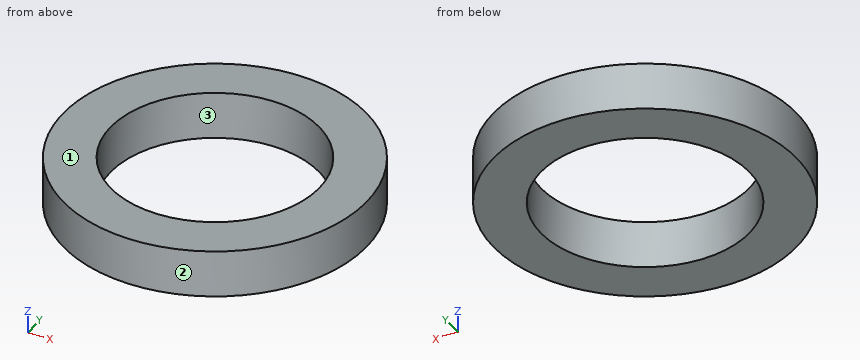
```python
from build123d import *

# Parameters (mm, degrees)
SKETCH1_R                = 2
BOSS_EXTRUDE1_DEPTH      = 6.35
CUT_EXTRUDE1_DEPTH       = 93.473426076
CUT_EXTRUDE1_DEPTH_BACK  = 93.473426076
SKETCH2_R                = 7
BOSS_EXTRUDE2_DEPTH      = 31.75
BOSS_EXTRUDE2_DEPTH_BACK = 12.7
SKETCH5_R                = 7
SKETCH6_R                = 7
BOSS_EXTRUDE3_DEPTH      = 6.35
FILLET1_R                = 6.35
FILLET2_R                = 3.175
SKETCH7_R                = 10.175
SKETCH7_R_2              = 7
BOSS_EXTRUDE4_DEPTH      = 3.175


with BuildPart() as part:
    # Sketch1 → Boss-Extrude1 (new, symmetric)
    # profile 1 of 3: a face of its own
    with BuildSketch(Plane.XY):
        Polygon((22.188571811, 51.670547503), (22.188571811, 37.229452497), (13.9055, 25.4), (13.9055, 0), (52.0055, 0), (52.0055, 25.4), (26.6055, 76.2), (13.9055, 76.2), (13.9055, 63.5), align=None)
        with Locations((33.493, 8.8)):
            Circle(SKETCH1_R, mode=Mode.SUBTRACT)
        with Locations((17.493, 8.8)):
            Circle(SKETCH1_R, mode=Mode.SUBTRACT)
    # profile 2 of 3: a face of its own
    with BuildSketch(Plane.XY):
        with Locations((17.493, 8.8)):
            Circle(SKETCH1_R)
    # profile 3 of 3: a face of its own
    with BuildSketch(Plane.XY):
        with Locations((33.493, 8.8)):
            Circle(SKETCH1_R)
    extrude(amount=BOSS_EXTRUDE1_DEPTH, both=True)

    # Sketch2 → Cut-Extrude1 (cut, two sides: drawn at the far end of the back side and taken through both)
    with BuildSketch(Plane.XY.offset(-CUT_EXTRUDE1_DEPTH_BACK)):
        with Locations((25.493, 16.8)):
            Circle(SKETCH2_R)
    extrude(amount=CUT_EXTRUDE1_DEPTH + CUT_EXTRUDE1_DEPTH_BACK, mode=Mode.SUBTRACT)

    # Fillet2
    fillet2_edges = [part.edges().sort_by_distance(p)[0] for p in [
        (22.188571811, 51.670547503, 0),
        (13.9055, 63.5, 0),
        (13.9055, 76.2, 0),
        (26.6055, 76.2, 0),
        (52.0055, 25.4, 0),
        (52.0055, 0, 0),
        (13.9055, 0, 0),
        (13.9055, 25.4, 0),
        (22.188571811, 37.229452497, 0),
    ]]
    fillet(fillet2_edges, radius=FILLET2_R)


with BuildPart() as body_2:
    # Sketch5 → Boss-Extrude2 (new, two sides: drawn at the far end of the back side and taken through both)
    with BuildSketch(Plane.XY.offset(6.35).offset(-BOSS_EXTRUDE2_DEPTH_BACK)):
        with Locations((25.493, 16.8)):
            Circle(SKETCH5_R)
    extrude(amount=BOSS_EXTRUDE2_DEPTH + BOSS_EXTRUDE2_DEPTH_BACK)


with BuildPart() as body_3:
    # Sketch6 → Boss-Extrude3 (new, symmetric)
    # profile 1 of 2: a face of its own
    with BuildSketch(Plane.XY.offset(15.875)):
        Polygon((0, -22.225), (0, 0), (-14.3805, 0), (-14.3805, 30.15), (-36.6055, 30.15), (-36.6055, -22.225), (-14.3805, -22.225), align=None)
        with Locations((-25.493, 16.8)):
            Circle(SKETCH6_R, mode=Mode.SUBTRACT)
    # profile 2 of 2: a face of its own
    with BuildSketch(Plane.XY.offset(15.875)):
        Polygon((14.3805, 30.15), (14.3805, 0), (0, 0), (0, -22.225), (14.3805, -22.225), (36.6055, -22.225), (36.6055, 30.15), align=None)
        with Locations((25.493, 16.8)):
            Circle(SKETCH6_R, mode=Mode.SUBTRACT)
    extrude(amount=BOSS_EXTRUDE3_DEPTH, both=True)

    # Fillet1
    fillet1_edges = [body_3.edges().sort_by_distance(p)[0] for p in [
        (-14.3805, 0, 15.875),
        (14.3805, 0, 15.875),
        (14.3805, 30.15, 15.875),
        (36.6055, 30.15, 15.875),
        (36.6055, -22.225, 15.875),
        (-36.6055, -22.225, 15.875),
        (-36.6055, 30.15, 15.875),
        (-14.3805, 30.15, 15.875),
    ]]
    fillet(fillet1_edges, radius=FILLET1_R)


with BuildPart() as body_4:
    # Sketch7 → Boss-Extrude4 (new body)
    with BuildSketch(Plane.XY.offset(6.35)):
        with Locations((25.493, 16.8)):
            Circle(SKETCH7_R)
        with Locations((25.493, 16.8)):
            Circle(SKETCH7_R_2, mode=Mode.SUBTRACT)
    extrude(amount=BOSS_EXTRUDE4_DEPTH)


solid = body_4.part
```
Model file for the job. Use its own axes, mm. Face numbers are marked on the shaded views. Coordinates: 2 decimals unless noted, no trailing zeros. Write each loop counter-clockwise with the first axis right and the second up, starting at its lowest first coordinate (ties: lowest second). Pieces come first, ordered by that corner, then holes. Notation, with made-up numbers: (85, -37.5) - (94, -37.5) arc R13 cw to (94, -14.5) - close; hole circle Ø4 at (47.25, 58.25). An arc over 180 degrees is marked (long way). Use a Markdown table: item, result. Add a question column.
Item 1: Band-saw the part on A-A, the plane y = 16.8. Write the cut outline in (x, z) (3 decimals), and give its area (3 significant figures).
Item 2: Two-plate mould, pull along X, no slides. Class the marked faces 1, 2 and 3: pulls with the +X half, pulls with the -X half, needs draft (parallel to the pull), parting line crosses it, or undercut.
Item 3: Drill centre lines: line 1 along Y through (x, z) = (25.5, 7.8) (3 decimals); line 2 along Y through (x, z) = (22.5, 8.1); line 3 along X through (y, z) = (15.25, 8.35). Where is each one in solid material? Low to high.
Item 4: Band-saw the part on D-D, the plane x = 18. Write the cut outline in (y, z) (3 decimals), and give its area (3 significant figures).
Item 5: Band-saw the part on C-C, the plane z = 7.95. Write the cut outline in (x, y) (3 decimals).
Item 6: Drop flat-ended pins along their axis: pin 1 (1.5 mm diameter, centred on y = 11, z = 6.5, fed in from +X); pin 2 (1 mm diameter, centred on x = 33, z = 8, fed in from -Y); pin 3 (1.5 mm diameter, centred on x = 24, z = 7.5, fed in from -Y). Give the stop position or say it passes through.
A:
| question | item | result |
|---|---|---|
| 1 | outline | (15.318, 6.35) - (18.493, 6.35) - (18.493, 9.525) - (15.318, 9.525) - close; (32.493, 6.35) - (35.668, 6.35) - (35.668, 9.525) - (32.493, 9.525) - close |
| 1 | area | 20.2 mm² |
| 2 | face 1 | needs draft |
| 2 | face 2 | parting line crosses it |
| 2 | face 3 | undercut |
| 3 | line 1 | y = 6.625 to 9.8, 23.8 to 26.975 |
| 3 | line 2 | y = 7.08 to 10.47, 23.13 to 26.52 |
| 3 | line 3 | x = 15.44 to 18.67, 32.32 to 35.55 |
| 4 | outline | (9.916, 6.35) - (23.684, 6.35) - (23.684, 9.525) - (9.916, 9.525) - close |
| 4 | area | 43.7 mm² |
| 5 | outline | circle Ø20.35 at (25.493, 16.8); hole circle Ø14 at (25.493, 16.8) |
| 6 | pin 1 | stops at x = 34.33 |
| 6 | pin 2 | stops at y = 9.42 |
| 6 | pin 3 | stops at y = 6.65 |
